Print and shaded views of the part. All mm, measured from the part's lowest x, y and z. Coordinates: 2 decimals unless noted, no trailing zeros. Order: outer loops, then holes, each group sorted by start corner. A loop starts at its lowest first (then second) coordinate and runs counter-clockwise, first axis right, second up.
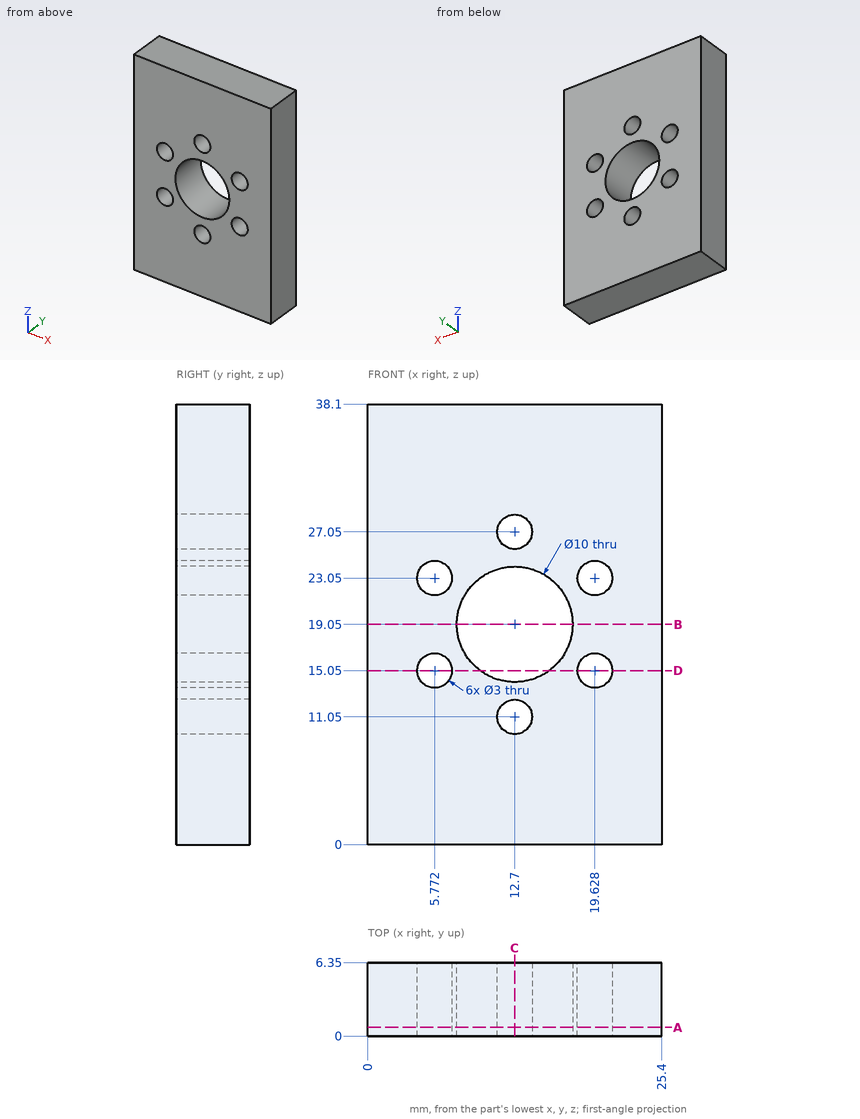
Q1. Cut at C-C, the plane x = 12.7. List the corners of the cut face in (y, z), plus the area to 3 significant figures.
Established:
outline: (0, 0) - (6.35, 0) - (6.35, 9.55) - (0, 9.55) - close; (0, 12.55) - (6.35, 12.55) - (6.35, 14.05) - (0, 14.05) - close; (0, 24.05) - (6.35, 24.05) - (6.35, 25.55) - (0, 25.55) - close; (0, 28.55) - (6.35, 28.55) - (6.35, 38.1) - (0, 38.1) - close
area: 140 mm2
Q2. Probe line 1 (Z direction, x = 12.7, y = 3.25); line 2 (Z direction, x = 19.5, y = 4.5); line 3 (Z direction, x = 14, y = 6). List the from-to ranges inside material, lowest first.
Established:
line 1: z = 0 to 9.55, 12.55 to 14.05, 24.05 to 25.55, 28.55 to 38.1
line 2: z = 0 to 13.56, 16.54 to 21.56, 24.54 to 38.1
line 3: z = 0 to 10.3, 11.8 to 14.22, 23.88 to 26.3, 27.8 to 38.1
Q3. Cut at B-B, the plane z = 19.05. List the corners of the cut face in (x, y), plus the area to 3 significant figures.
Established:
outline: (0, 0) - (7.7, 0) - (7.7, 6.35) - (0, 6.35) - close; (17.7, 0) - (25.4, 0) - (25.4, 6.35) - (17.7, 6.35) - close
area: 97.8 mm2
Q4. Cut at A-A, the plane y = 0.75. List the corners of the cut face in (x, z), plus the area to 3 significant figures.
Established:
outline: (0, 0) - (25.4, 0) - (25.4, 38.1) - (0, 38.1) - close; hole circle Ø3 at (5.77, 15.05); hole circle Ø3 at (5.77, 23.05); hole circle Ø10 at (12.7, 19.05); hole circle Ø3 at (12.7, 11.05); hole circle Ø3 at (12.7, 27.05); hole circle Ø3 at (19.63, 15.05); hole circle Ø3 at (19.63, 23.05)
area: 847 mm2
Q5. Cut at D-D, the plane z = 15.05. List the corners of the cut face in (x, y), plus the area to 3 significant figures.
Established:
outline: (0, 0) - (4.27, 0) - (4.27, 6.35) - (0, 6.35) - close; (7.27, 0) - (9.7, 0) - (9.7, 6.35) - (7.27, 6.35) - close; (15.7, 0) - (18.13, 0) - (18.13, 6.35) - (15.7, 6.35) - close; (21.13, 0) - (25.4, 0) - (25.4, 6.35) - (21.13, 6.35) - close
area: 85.1 mm2
